from build123d import *

# Parameters (mm, degrees)
SKETCH1_W           = 254.5
SKETCH1_H           = 172
BOSS_EXTRUDE1_DEPTH = 1
SKETCH2_W           = 230
SKETCH2_H           = 148
BOSS_EXTRUDE2_DEPTH = 9
SKETCH3_R           = 1.75
CUT_EXTRUDE1_DEPTH  = 2
SKETCH4_W           = 217.5
SKETCH4_H           = 135
CUT_EXTRUDE2_DEPTH  = 0.1


with BuildPart() as part:
    # Sketch1 → Boss-Extrude1 (new body)
    with BuildSketch(Plane.XY):
        Rectangle(SKETCH1_W, SKETCH1_H)
    extrude(amount=BOSS_EXTRUDE1_DEPTH)

    # Sketch2 → Boss-Extrude2 (add)
    with BuildSketch(Plane(origin=(0, 0, 0), x_dir=(-1, 0, 0), z_dir=(0, 0, -1))):
        with Locations((0, -2.5)):
            Rectangle(SKETCH2_W, SKETCH2_H)
    extrude(amount=BOSS_EXTRUDE2_DEPTH)

    # Sketch3 → Cut-Extrude1 (cut)
    with BuildSketch(Plane(origin=(0, 0, -9), x_dir=(-1, 0, 0), z_dir=(0, 0, -1))):
        with Locations((29, -26.5)):
            Circle(SKETCH3_R)
        with Locations((-29, -26.5)):
            Circle(SKETCH3_R)
        with Locations((-29, 22.5)):
            Circle(SKETCH3_R)
        with Locations((29, 22.5)):
            Circle(SKETCH3_R)
    extrude(amount=-CUT_EXTRUDE1_DEPTH, mode=Mode.SUBTRACT)

    # Sketch4 → Cut-Extrude2 (cut)
    with BuildSketch(Plane.XY.offset(1)):
        Rectangle(SKETCH4_W, SKETCH4_H)
    extrude(amount=-CUT_EXTRUDE2_DEPTH, mode=Mode.SUBTRACT)


solid = part.part
Read the model definition and answer for the solid it produces. Units are mm, in the model's axes. A direction names the side the tool comes from. Round coordinates to 2 decimals unless told otherwise and drop trailing zeros. Loops run counter-clockwise (first coordinate to the right, second up) from the corner with the lowest first, then second, coordinate; pieces in that order, holes last.
Q1. Which of the six approach directions +Z, -Z, +X, -X, +Y, -Y give full straight-line access (tool end or side, diameter ignored) to faces 1 (the face through (2, 71.5, -4)), 2 (the face through (-115, -4, -4)), 3 (the face through (2, -76.5, -4))?
Q2. Each of these flat-tipped pins is pushed along its axis until it touches: pin 1 (3 mm diameter, centred on x = 29, y = -26.5, fed in from +Z); pin 2 (4.5 mm diameter, centred on y = 31, z = -3.5, fed in from +X); pin 3 (6 mm diameter, centred on y = 55.5, z = -2.5, fed in from -X); pin 4 (4 mm diameter, centred on x = 98.5, z = -2.5, fed in from -Y). Where does it stop, or does it pass through?
Q3. Section B-B on x = -5 is taken. Write down the section's boundary in (y, z), and give its area (3 significant figures).
Q4. Consider probe 1 along Y at (x, z) = (-29, -8.1); probe 2 along Y at (x, z) = (91.5, -4.25); probe 3 along Z at (x, y) = (-11.5, -9). Determine where each line is inside the solid, lowest interval first.
Q5. Section C-C on z = -2.25 is taken. Write down the section's boundary in (x, y).
Q6. Section A-A on y = 4 is taken. Write down the section's boundary in (x, z).
Output:
1. face 1: -Z, +X, -X, +Y
1. face 2: -Z, -X, +Y, -Y
1. face 3: -Z, +X, -X, -Y
2. pin 1: stops at z = 0.9
2. pin 2: stops at x = 115
2. pin 3: stops at x = -127.25
2. pin 4: stops at y = -76.5
3. outline: (-86, 0) - (-76.5, 0) - (-76.5, -9) - (71.5, -9) - (71.5, 0) - (86, 0) - (86, 1) - (67.5, 1) - (67.5, 0.9) - (-67.5, 0.9) - (-67.5, 1) - (-86, 1) - close
3. area: 1,490 mm2
4. probe 1: y = -76.5 to -28.25, -24.75 to 20.75, 24.25 to 71.5
4. probe 2: y = -76.5 to 71.5
4. probe 3: z = -9 to 0.9
5. outline: (-115, -76.5) - (115, -76.5) - (115, 71.5) - (-115, 71.5) - close
6. outline: (-127.25, 0) - (-115, 0) - (-115, -9) - (115, -9) - (115, 0) - (127.25, 0) - (127.25, 1) - (108.75, 1) - (108.75, 0.9) - (-108.75, 0.9) - (-108.75, 1) - (-127.25, 1) - close
